```python
from build123d import *

# Parameters (mm, degrees)
BOSS_EXTRUDE1_DEPTH  = 6
CUT_EXTRUDE1_DEPTH   = 6
M5_CLEARANCE_HOLE1_D = 5.3
CUT_EXTRUDE2_DEPTH   = 22
M5_CLEARANCE_HOLE2_D = 5.3
CUT_EXTRUDE3_DEPTH   = 6
CUT_EXTRUDE4_DEPTH   = 6


with BuildPart() as part:
    # Sketch2 → Boss-Extrude1 (new body)
    with BuildSketch(Plane.XY):
        with BuildLine():
            Line((-55, -80), (55, -80))
            ThreePointArc((55, -80), (58.535533906, -78.535533906), (60, -75))
            Line((60, -75), (60, 75))
            ThreePointArc((60, 75), (58.535533906, 78.535533906), (55, 80))
            Line((55, 80), (-55, 80))
            ThreePointArc((-55, 80), (-58.535533906, 78.535533906), (-60, 75))
            Line((-60, 75), (-60, -75))
            ThreePointArc((-60, -75), (-58.535533906, -78.535533906), (-55, -80))
        make_face()
    extrude(amount=BOSS_EXTRUDE1_DEPTH)

    # Sketch3 → Cut-Extrude1 (cut)
    with BuildSketch(Plane.XY.offset(6)):
        with BuildLine():
            Line((2.54, -17.5), (2.54, -62.5))
            ThreePointArc((2.54, -62.5), (0, -65.04), (-2.54, -62.5))
            Line((-2.54, -62.5), (-2.54, -17.5))
            ThreePointArc((-2.54, -17.5), (0, -14.96), (2.54, -17.5))
        make_face()
    extrude(amount=-CUT_EXTRUDE1_DEPTH, mode=Mode.SUBTRACT)

    # M5 Clearance Hole1 (through all)
    with Locations(Plane.XY.offset(6)):
        with Locations((-23.57, -63.57), (-23.57, -16.43), (23.57, -16.43), (23.57, -63.57)):
            Hole(M5_CLEARANCE_HOLE1_D / 2)

    # Sketch6 → Cut-Extrude2 (cut)
    with BuildSketch(Plane.XY.offset(6)):
        with BuildLine():
            Line((-32.03, -16.43), (-32.03, -23.43))
            ThreePointArc((-32.03, -23.43), (-34.57, -25.97), (-37.11, -23.43))
            Line((-37.11, -23.43), (-37.11, -16.43))
            ThreePointArc((-37.11, -16.43), (-34.57, -13.89), (-32.03, -16.43))
        make_face()
    cut_extrude2 = extrude(amount=-CUT_EXTRUDE2_DEPTH, mode=Mode.SUBTRACT)

    # M5 Clearance Hole2 (through all)
    with Locations(Plane.XY.offset(6)):
        with Locations((-34.57, 41.47)):
            m5_clearance_hole2 = Hole(M5_CLEARANCE_HOLE2_D / 2)

    # Sketch9 → Cut-Extrude3 (cut)
    with BuildSketch(Plane.XY.offset(6)):
        with BuildLine():
            Line((-47.03, 25.07), (-47.03, -64.93))
            ThreePointArc((-47.03, -64.93), (-49.57, -67.47), (-52.11, -64.93))
            Line((-52.11, -64.93), (-52.11, 25.07))
            ThreePointArc((-52.11, 25.07), (-49.57, 27.61), (-47.03, 25.07))
        make_face()
    cut_extrude3 = extrude(amount=-CUT_EXTRUDE3_DEPTH, mode=Mode.SUBTRACT)

    # Mirror2: Cut-Extrude2, M5 Clearance Hole2, Cut-Extrude3 across plane
    add(cut_extrude2.mirror(Plane(origin=(0, 0, 0), x_dir=(0, 0, 1), z_dir=(1, 0, 0))), mode=Mode.SUBTRACT)
    add(m5_clearance_hole2.mirror(Plane(origin=(0, 0, 0), x_dir=(0, 0, 1), z_dir=(1, 0, 0))), mode=Mode.SUBTRACT)
    add(cut_extrude3.mirror(Plane(origin=(0, 0, 0), x_dir=(0, 0, 1), z_dir=(1, 0, 0))), mode=Mode.SUBTRACT)

    # Sketch11 → Cut-Extrude4 (cut)
    with BuildSketch(Plane.XY.offset(6)):
        with BuildLine():
            Line((-7.46, 68.5), (-7.46, 61.5))
            ThreePointArc((-7.46, 61.5), (-10, 58.96), (-12.54, 61.5))
            Line((-12.54, 61.5), (-12.54, 68.5))
            ThreePointArc((-12.54, 68.5), (-10, 71.04), (-7.46, 68.5))
        make_face()
        with BuildLine():
            Line((12.54, 68.5), (12.54, 61.5))
            ThreePointArc((12.54, 61.5), (10, 58.96), (7.46, 61.5))
            Line((7.46, 61.5), (7.46, 68.5))
            ThreePointArc((7.46, 68.5), (10, 71.04), (12.54, 68.5))
        make_face()
    extrude(amount=-CUT_EXTRUDE4_DEPTH, mode=Mode.SUBTRACT)


solid = part.part
```
For this review, take the finished solid that the model builds, in its own axes (mm). A direction names the side the tool comes from. Coordinates: 2 decimals unless noted, no trailing zeros. Order: outer loops, then holes, each group sorted by start corner. A loop starts at its lowest first (then second) coordinate and runs counter-clockwise, first axis right, second up. Notation, with made-up numbers: (66.25, 79) -> (74.25, 79) arc R35 ccw to (74.25, 116) -> close; hole circle Ø7 at (13.25, 84.25). An arc over 180 degrees is marked (long way). Use CSV: the item, a comma, the result in double quotes. Start each with the question number.
Item 1: Wall thickness on probe 1 along Y at (x, z) = (23.57, 4); probe 2 along X at (y, z) = (-52, 4.9); probe 3 along Y at (x, z) = (-34.57, 2.8): over which ranges is each line inside the solid? List them lowest first.
Item 2: We need section D-D, the plane x = -23.57. Give the boundary of the cut face in (y, z), then the cut area to 3 significant figures.
Item 3: We need section B-B, the plane x = -10. Give the boundary of the cut face in (y, z).
Item 4: We need section A-A, the plane y = 23. Give the boundary of the cut face in (x, z), then the cut area to 3 significant figures.
Item 5: Insertion check: pin 1 (6 mm diameter, centred on x = 23.57, y = -16.43, fed in from -Z); pin 2 (4 mm diameter, centred on x = 34.57, y = 41.47, fed in from +Z). Each pin has a flat end and moves straight along its axis. Give the tip position at first contact, or say it passes through.
Item 6: Draft analysis for pull direction X (two halves, no side actions). For faces 1 (the face through (23.91, -60.94, 2.96)), 2 (the face through (-60, 1, 3)), 3 (the face through (-37.11, -20, 3)), 4 (the face through (-1, 1, 6)), state which applies: pulls with the +X half, pulls with the -X half, needs draft (parallel to the pull), parting line crosses it, or undercut.
Item 7: We need section C-C, the plane y = -44.5. Give the boundary of the cut face in (x, z), then the cut area to 3 significant figures.
Item 8: For faces 5 (the face through (59, 78, 3)), 6 (the face through (49.63, 27.61, 3.04)), list the 3-axis set-ups (+Z, -Z, +X, -X, +Y, -Y) from which the entire face can be reached by the end or side of a thin tool; tool diameter is ignored.
Derived:
1,probe 1,"y = -80 to -66.22, -60.92 to -19.08, -13.78 to 80"
1,probe 2,"x = -60 to -52.11, -47.03 to -2.54, 2.54 to 47.03, 52.11 to 60"
1,probe 3,"y = -80 to -25.97, -13.89 to 38.82, 44.12 to 80"
2,outline,"(-80, 0) -> (-66.22, 0) -> (-66.22, 6) -> (-80, 6) -> close; (-60.92, 0) -> (-19.08, 0) -> (-19.08, 6) -> (-60.92, 6) -> close; (-13.78, 0) -> (80, 0) -> (80, 6) -> (-13.78, 6) -> close"
2,area,"896 mm^2"
3,outline,"(-80, 0) -> (58.96, 0) -> (58.96, 6) -> (-80, 6) -> close; (71.04, 0) -> (80, 0) -> (80, 6) -> (71.04, 6) -> close"
4,outline,"(-60, 0) -> (-52.11, 0) -> (-52.11, 6) -> (-60, 6) -> close; (-47.03, 0) -> (47.03, 0) -> (47.03, 6) -> (-47.03, 6) -> close; (52.11, 0) -> (60, 0) -> (60, 6) -> (52.11, 6) -> close"
4,area,"659 mm^2"
5,pin 1,"stops at z = 0"
5,pin 2,"passes through"
6,face 1,"undercut"
6,face 2,"pulls with the -X half"
6,face 3,"undercut"
6,face 4,"needs draft"
7,outline,"(-60, 0) -> (-52.11, 0) -> (-52.11, 6) -> (-60, 6) -> close; (-47.03, 0) -> (-2.54, 0) -> (-2.54, 6) -> (-47.03, 6) -> close; (2.54, 0) -> (47.03, 0) -> (47.03, 6) -> (2.54, 6) -> close; (52.11, 0) -> (60, 0) -> (60, 6) -> (52.11, 6) -> close"
7,area,"629 mm^2"
8,face 5,"+Z, -Z, +X, +Y"
8,face 6,"+Z, -Z"
